Work out the finished part from the listing and answer in its coordinate system (mm). Round coordinates to 2 decimals unless told otherwise and drop trailing zeros. Write each loop counter-clockwise with the first axis right and the second up, starting at its lowest first coordinate (ties: lowest second). Pieces come first, ordered by that corner, then holes.
Autodesk Inventor part; units mm, degrees
ref_plane "YZ Plane" through (0, 0, 0) normal (1, 0, 0) x (0, 1, 0)
ref_plane "XZ Plane" through (0, 0, 0) normal (0, 1, 0) x (-1, 0, 0)
ref_plane "XY Plane" through (0, 0, 0) normal (0, 0, 1) x (1, 0, 0)
sketch "Sketch1" plane through (0, 0, 0) normal (0, 0, 1) x (1, 0, 0)
  line L0 (0, 0) -> (152.4, 0)
  line L1 (152.4, 0) -> (152.4, 76.2)
  line L2 (152.4, 76.2) -> (0, 76.2)
  line L3 (0, 76.2) -> (0, 0)
  dimension "d0" = 152.4
  dimension "d1" = 76.2
extrude "Extrusion1" add sketch "Sketch1" along normal blind 3.175
sketch "Sketch2" plane through (0, 0, 3.175) normal (0, 0, 1) x (1, 0, 0)
  line L0 (152.4, 76.2) -> (0, 76.2)
  line L1 (0, 76.2) -> (0, 0)
  circle A0 centre (52.3875, 36.5125) radius 2.8067
  circle A1 centre (100.0125, 36.5125) radius 2.8067
  circle A2 centre (19.05, 36.5125) radius 2.8067
  circle A3 centre (133.35, 36.5125) radius 2.8067
  circle A4 centre (76.2, 36.5125) radius 14.2875
  line L2 (0, 0) -> (152.4, 0)
  dimension "d8" = 5.6134
  dimension "d9" = 5.6134
  dimension "d11" = 5.6134
  dimension "d12" = 5.6134
  dimension "d22" = 28.575
  dimension "d23" = 76.2
  dimension "d24" = 36.5125
  dimension "d25" = 36.5125
  dimension "d26" = 36.5125
  dimension "d27" = 36.5125
  dimension "d28" = 36.5125
extrude "Extrusion3" cut sketch "Sketch2" against normal blind 25.4
fillet "Fillet2" radius 6.35 4 edges at (152.4, 0, 1.5875) (152.4, 76.2, 1.5875) (0, 76.2, 1.5875) (0, 0, 1.5875)
properties part number "GearboxPlate" material "Aluminum 6061"
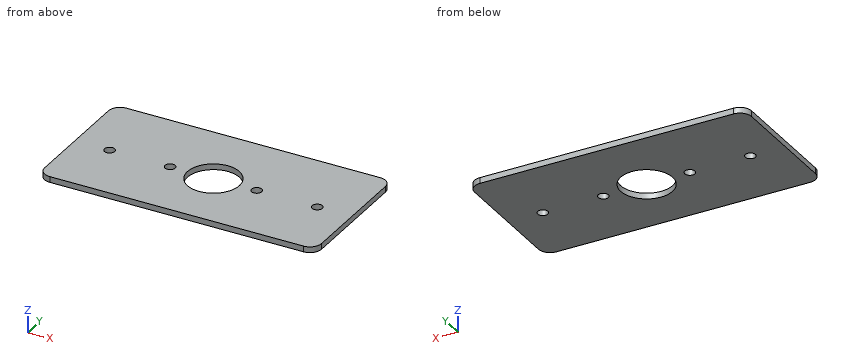
Q1. Find section A-A (x = 76.2). Determine the outline of the cut face in (y, z) (3 decimals), plus the area to 3 significant figures.
Q2. Find section C-C (x = 19.05). Determine the outline of the cut face in (y, z) (3 decimals).
Q3. Find the intervals of material crossed by L1, parallel to Y at x = 133, z = 1.45; L2, parallel to X at y = 35, z = 2.35; L3, parallel to Y at x = 76.2, z = 1.9 (3 decimals), in increasing order.
Q4. Given pin 1 (3.5 mm diameter, centred on x = 52.39, y = 36.51, fed in from -Z), flat-ended and moving along its own axis, determine where the tip first touches the part or whether it passes through.
Q5. Find section B-B (z = 0.9). Count the separate pieces of the cut face and the enclosed holes in it, plus the area to 3 significant figures.
Report:
1. outline: (0, 0) - (22.225, 0) - (22.225, 3.175) - (0, 3.175) - close; (50.8, 0) - (76.2, 0) - (76.2, 3.175) - (50.8, 3.175) - close
1. area: 151 mm2
2. outline: (0, 0) - (33.706, 0) - (33.706, 3.175) - (0, 3.175) - close; (39.319, 0) - (76.2, 0) - (76.2, 3.175) - (39.319, 3.175) - close
3. L1: y = 0 to 33.73, 39.3 to 76.2
3. L2: x = 0 to 16.69, 21.41 to 50.02, 54.75 to 61.99, 90.41 to 97.65, 102.38 to 130.99, 135.71 to 152.4
3. L3: y = 0 to 22.225, 50.8 to 76.2
4. pin 1: passes through
5. separate pieces: 1
5. enclosed holes: 5
5. area: 10,800 mm2
